Geometry: final body of the model. Coordinates: model frame, mm. A direction names the side the tool comes from. Give positions to 0.01 mm unless a question says otherwise; leave off trailing zeros. Order: outer loops, then holes, each group sorted by start corner. A loop starts at its lowest first (then second) coordinate and runs counter-clockwise, first axis right, second up. Notation, with made-up numbers: (48.25, 12.5) - (78.25, 12.5) arc R17 cw to (78.25, 44.5) - close; hole circle Ø9 at (46, -21.5). An arc over 180 degrees is marked (long way). Put each result on its own line as item: value. Start each with the question number.
1. Section A-A on z = 1. Return the cut outline in (x, y).
2. Mould query, pull axis X, two halves, no side actions, for faces 1 (the flat face through (0, 7, 2.4)), 2 (the flat face through (7.324, 0, -4)), 3 (the flat face through (0, -14.4, 5)). Classes: pulls with the +X half, pulls with the -X half, needs draft (parallel to the pull), parting line crosses it, or undercut.
3. Set-up query: faces 4 (the flat face through (-1.2, 19, 1)), 5 (the flat face through (-2, 17, 2.4)), 6 (the flat face through (-2, -17, 2.4)). Return all of +Z, -Z, +X, -X, +Y, -Y with unobstructed straight access to the full face (end or side cutting, diameter ignored); none if empty.
4. Ray query, line 1 along Y through (x, z) = (-1.5, -14.5); line 2 along Z through (x, y) = (-3.75, -8.5); line 3 along Y through (x, z) = (0, 5.5). Return the intervals inside material, ascending. Write a range as from..to.
5. Section B-B on y = 6.6. Return the cut outline in (x, z).
6. First-contact query: P1, Ø5, axis at x = 5, z = 7.5, coming from the -Y side; P2, Ø6.5, axis at x = 0, y = 18.5, coming from the +Z side; P3, Ø0.7, axis at y = 0, z = 13, coming from the +X side. Flat tips, straight axial feed; report the tip coordinate or a pass-through.
7. Section D-D on y = -6. Return the cut outline in (x, z).
8. Section C-C on x = -3.75. Return the cut outline in (y, z).
from build123d import *

# Parameters (mm, degrees)
BOSS_EXTRU_2_DEPTH      = 2.4
ESQUISSE3_W             = 14.64741017
ESQUISSE3_H             = 28.8
BOSS_EXTRU_3_DEPTH      = 4.8
BOSS_EXTRU_4_DEPTH      = 4.8
ESQUISSE7_R             = 3
BOSS_EXTRU_5_DEPTH      = 7.2
ENL_V_START             = -4.8
ESQUISSE8_R             = 3
ENL_V_MAT_EXTRU_1_DEPTH = 4.8
ESQUISSE9_W             = 14.64741017
ESQUISSE9_H             = 28.8
BOSS_EXTRU_6_DEPTH      = 19.2
CONG_1_R                = 1


with BuildPart() as part:
    # Esquisse1 → Boss.-Extru.2 (new body)
    with BuildSketch(Plane.XY):
        with BuildLine():
            Line((-7.323705085, 20.4), (-1.2, 20.4))
            Line((-1.2, 20.4), (-1.2, 16.8))
            ThreePointArc((-1.2, 16.8), (0, 15.6), (1.2, 16.8))
            Line((1.2, 16.8), (1.2, 20.4))
            Line((1.2, 20.4), (7.323705085, 20.4))
            Line((7.323705085, 20.4), (7.323705085, -20.4))
            Line((7.323705085, -20.4), (1.2, -20.4))
            Line((1.2, -20.4), (1.2, -16.8))
            ThreePointArc((1.2, -16.8), (0, -15.6), (-1.2, -16.8))
            Line((-1.2, -16.8), (-1.2, -20.4))
            Line((-1.2, -20.4), (-7.323705085, -20.4))
            Line((-7.323705085, -20.4), (-7.323705085, 20.4))
        make_face()
    extrude(amount=BOSS_EXTRU_2_DEPTH)

    # Esquisse3 → Boss.-Extru.3 (add)
    with BuildSketch(Plane.XY.offset(2.4)):
        Rectangle(ESQUISSE3_W, ESQUISSE3_H)
    extrude(amount=BOSS_EXTRU_3_DEPTH)

    # Esquisse4 → Boss.-Extru.4 (add)
    with BuildSketch(Plane.XY.offset(7.2)):
        with BuildLine():
            Line((0, 12), (0, 14.4))
            ThreePointArc((8e-09, 14.4), (-4.466852593, 12.994312153), (-7.323705085, 9.283904587))
            Line((-7.323705085, 9.283904587), (-7.323705085, 3.916095413))
            ThreePointArc((-7.323705085, 3.916095413), (-5.741131727, 1.319904689), (-3.286183333, -0.473966292))
            Line((-3.286183333, -0.473966292), (-3.286183333, -3.414033708))
            ThreePointArc((-3.286183333, -3.414033708), (-1.958044771, -4.964937052), (0, -5.544))
            Line((0, -5.544), (0, -3.744))
            ThreePointArc((0, -3.744), (-0.763253879, -3.574166714), (-1.382478965, -3.096715017))
            Line((-1.382478965, -3.096715017), (-1.382478965, 1.379966292))
            ThreePointArc((-1.382478965, 1.379966292), (-5.354819419, 7.297071724), (0, 12))
        make_face()
        with BuildLine():
            ThreePointArc((7.323705085, 9.283904587), (4.466852599, 12.994312149), (8e-09, 14.4))
            Line((0, 14.4), (0, 12))
            ThreePointArc((0, 12), (5.354819419, 7.297071724), (1.382478965, 1.379966292))
            Line((1.382478965, 1.379966292), (1.382478965, -3.096715017))
            ThreePointArc((1.382478965, -3.096715017), (0.763253879, -3.574166714), (0, -3.744))
            Line((0, -3.744), (0, -5.544))
            ThreePointArc((0, -5.544), (1.920803148, -4.988752086), (3.249094107, -3.49428626))
            Line((3.249094107, -3.49428626), (3.286183333, -0.473966292))
            ThreePointArc((3.286183333, -0.473966292), (5.741131727, 1.319904689), (7.323705085, 3.916095413))
            Line((7.323705085, 3.916095413), (7.323705085, 9.283904587))
        make_face()
    extrude(amount=BOSS_EXTRU_4_DEPTH)

    # Esquisse7 → Boss.-Extru.5 (add)
    with BuildSketch(Plane.XY.offset(7.2)):
        with BuildLine():
            Line((-1.382478965, 1.379966292), (-1.382478965, -3.096715017))
            ThreePointArc((-1.382478965, -3.096715017), (0, -3.744), (1.382478965, -3.096715017))
            Line((1.382478965, -3.096715017), (1.382478965, 1.379966292))
            ThreePointArc((1.382478965, 1.379966292), (0, 12), (-1.382478965, 1.379966292))
        make_face()
        with Locations((0, 6.6)):
            Circle(ESQUISSE7_R, mode=Mode.SUBTRACT)
    extrude(amount=BOSS_EXTRU_5_DEPTH)

    # Esquisse8 → Enlèv. mat.-Extru.1 (cut)
    with BuildSketch(Plane.XY.offset(7.2).offset(ENL_V_START)):
        with Locations((0, 6.6)):
            Circle(ESQUISSE8_R)
    extrude(amount=ENL_V_MAT_EXTRU_1_DEPTH, mode=Mode.SUBTRACT)

    # Esquisse9 → Boss.-Extru.6 (add)
    with BuildSketch(Plane(origin=(0, 0, 0), x_dir=(-1, 0, 0), z_dir=(0, 0, -1))):
        Rectangle(ESQUISSE9_W, ESQUISSE9_H)
    extrude(amount=BOSS_EXTRU_6_DEPTH)

    # Congé1
    cong_1_edges = [part.edges().sort_by_distance(p)[0] for p in [
        (7.323705085, 20.4, 1.2),
        (7.323705085, -20.4, 1.2),
        (-7.323705085, -20.4, 1.2),
        (-7.323705085, 20.4, 1.2),
    ]]
    fillet(cong_1_edges, radius=CONG_1_R)


solid = part.part
Resolved:
1. outline: (-7.32, -19.4) arc R1 ccw to (-6.32, -20.4) - (-1.2, -20.4) - (-1.2, -16.8) arc R1.2 cw to (1.2, -16.8) - (1.2, -20.4) - (6.32, -20.4) arc R1 ccw to (7.32, -19.4) - (7.32, 19.4) arc R1 ccw to (6.32, 20.4) - (1.2, 20.4) - (1.2, 16.8) arc R1.2 cw to (-1.2, 16.8) - (-1.2, 20.4) - (-6.32, 20.4) arc R1 ccw to (-7.32, 19.4) - close
2. face 1: undercut
2. face 2: pulls with the +X half
2. face 3: needs draft
3. face 4: +Z, -Z, +Y
3. face 5: +Z, +X, -X, +Y
3. face 6: +Z, +X, -X, -Y
4. line 1: -14.4..14.4
4. line 2: -19.2..7.2
4. line 3: -14.4..3.6, 9.6..14.4
5. outline: (-7.32, -19.2) - (7.32, -19.2) - (7.32, 12) - (5.4, 12) - (5.4, 14.4) - (3, 14.4) - (3, 2.4) - (-3, 2.4) - (-3, 14.4) - (-5.4, 14.4) - (-5.4, 12) - (-7.32, 12) - close
6. P1: y = -14.4
6. P2: z = 2.4
6. P3: x = 1.38
7. outline: (-7.32, -19.2) - (7.32, -19.2) - (7.32, 7.2) - (-7.32, 7.2) - close
8. outline: (-20.4, 0) - (-14.4, 0) - (-14.4, -19.2) - (14.4, -19.2) - (14.4, 0) - (20.4, 0) - (20.4, 2.4) - (14.4, 2.4) - (14.4, 7.2) - (13.44, 7.2) - (13.44, 12) - (10.49, 12) - (10.49, 14.4) - (2.71, 14.4) - (2.71, 12) - (-0.24, 12) - (-0.24, 7.2) - (-14.4, 7.2) - (-14.4, 2.4) - (-20.4, 2.4) - close
